from build123d import *

# Parameters (mm, degrees)
SKETCH2_W           = 48.13
SKETCH2_H           = 41.71
BOSS_EXTRUDE1_DEPTH = 1.71
SKETCH3_R           = 1.5
CUT_EXTRUDE1_DEPTH  = 10.71
CUT_EXTRUDE2_DEPTH  = 10.71
FILLET3_R           = 2.5
SKETCH8_W           = 8.21
SKETCH8_H           = 30.23
BOSS_EXTRUDE2_DEPTH = 10.03


with BuildPart() as part:
    # Sketch2 → Boss-Extrude1 (new body)
    with BuildSketch(Plane(origin=(0, 0, 0), x_dir=(1, 0, 0), z_dir=(0, 1, 0))):
        Rectangle(SKETCH2_W, SKETCH2_H)
    extrude(amount=BOSS_EXTRUDE1_DEPTH)

    # Sketch3 → Cut-Extrude1 (cut)
    with BuildSketch(Plane(origin=(0, 1.71, 0), x_dir=(1, 0, 0), z_dir=(0, 1, 0))):
        with Locations(Location((-21.545702182, 18.174313444, 0), (0, 0, 270))):
            Circle(SKETCH3_R)
    cut_extrude1 = extrude(amount=-CUT_EXTRUDE1_DEPTH, mode=Mode.SUBTRACT)

    # Sketch4 → Cut-Extrude2 (cut)
    with BuildSketch(Plane(origin=(0, 1.71, 0), x_dir=(1, 0, 0), z_dir=(0, 1, 0))):
        with BuildLine():
            ThreePointArc((-20.045702182, -18.175), (-20.485042011, -17.114339828), (-21.545702182, -16.675))
            Line((-21.545702182, -16.675), (-21.545702182, -18.175))
            Line((-21.545702182, -18.175), (-21.545702182, -19.675))
            ThreePointArc((-21.545702182, -19.675), (-20.485042011, -19.235660172), (-20.045702182, -18.175))
        make_face()
        with BuildLine():
            Line((-21.545702182, -18.175), (-21.545702182, -16.675))
            ThreePointArc((-21.545702182, -16.675), (-23.045702182, -18.175), (-21.545702182, -19.675))
            Line((-21.545702182, -19.675), (-21.545702182, -18.175))
        make_face()
    cut_extrude2 = extrude(amount=-CUT_EXTRUDE2_DEPTH, mode=Mode.SUBTRACT)

    # Fillet3
    fillet3_edges = [part.edges().sort_by_distance(p)[0] for p in [
        (24.065, 0.855, 20.855),
        (-24.065, 0.855, 20.855),
        (-24.065, 0.855, -20.855),
        (24.065, 0.855, -20.855),
    ]]
    fillet(fillet3_edges, radius=FILLET3_R)

    # Mirror1: Cut-Extrude1, Cut-Extrude2 across plane
    add(cut_extrude1.mirror(Plane(origin=(0, 0, 0), x_dir=(0, 0, 1), z_dir=(1, 0, 0))), mode=Mode.SUBTRACT)
    add(cut_extrude2.mirror(Plane(origin=(0, 0, 0), x_dir=(0, 0, 1), z_dir=(1, 0, 0))), mode=Mode.SUBTRACT)

    # Sketch8 → Boss-Extrude2 (add)
    with BuildSketch(Plane(origin=(0, 1.71, 0), x_dir=(1, 0, 0), z_dir=(0, 1, 0))):
        with Locations((-19.96, 0)):
            Rectangle(SKETCH8_W, SKETCH8_H)
    extrude(amount=BOSS_EXTRUDE2_DEPTH)


solid = part.part
The listing builds one solid part. Answer for the finished solid, in the listing's coordinates (mm). A direction names the side the tool comes from. Round coordinates to 2 decimals unless told otherwise and drop trailing zeros. Order: outer loops, then holes, each group sorted by start corner. A loop starts at its lowest first (then second) coordinate and runs counter-clockwise, first axis right, second up. Notation, with made-up numbers: M 8.5,-21 L 35.5,-21 A18 cw 35.5,-13 Z; hole C -35.75,86 d9. An arc over 180 degrees is marked long. Answer in a Markdown table with one row per item. Add a question column.
1) The part is cut by section B-B on z = 13. Determine the outline of the cut face in (x, y) (3 decimals).
2) The part is cut by section A-A on x = -21. Determine the outline of the cut face in (y, z) (3 decimals), plus the area to 3 significant figures.
3) The part is cut by section D-D on x = 12.5. Determine the outline of the cut face in (y, z) (3 decimals).
4) Flat-ended cylindrical pins translate along their axes: pin 1 Ø5 at (x, z) = (21.55, -18.17) entering from +Y; pin 2 Ø6 at (y, z) = (4.5, 12) entering from +X (3 decimals); pin 3 Ø2.5 at (x, z) = (-21.55, -18.17) entering from +Y; pin 4 Ø2.5 at (x, y) = (-18, 5.5) entering from +Z (3 decimals). Find the tip coordinate at first contact, or state that the pin passes through.
5) The part is cut by section C-C on y = 7.25. Determine the outline of the cut face in (x, z) (3 decimals), plus the area to 3 significant figures.
6) Consider line 1 along Z through (x, y) = (-20.5, 1.5) (3 decimals); line 2 along Y through (x, z) = (17, -4); line 3 along X through (y, z) = (2, -15) (3 decimals). Determine where each line is inside the solid, lowest interval first. Write a range as from..to.
7) Determine the mould class of faces 1 (the face through (0, 0, 0)), 2 (the face through (0, 1, 20.855)), 3 (the face through (-21.48, 0.867, -19.673)) for opening direction Z: pulls with the +Z half, pulls with the -Z half, needs draft (parallel to the pull), parting line crosses it, or undercut.
8) Which of the six approach directions +Z, -Z, +X, -X, +Y, -Y give full straight-line access (tool end or side, diameter ignored) to faces 4 (the face through (-15.855, 7, 0)), 5 (the face through (-20, 7, 15.115)), 6 (the face through (-20, 7, -15.115))?
Findings below:
| question | item | result |
|---|---|---|
| 1 | outline | M -24.065,0 L 24.065,0 L 24.065,1.71 L -15.855,1.71 L -15.855,11.74 L -24.065,11.74 Z |
| 2 | outline | M 0,-20.855 L 1.71,-20.855 L 1.71,-19.572 L 0,-19.572 Z; M 0,-16.777 L 1.71,-16.777 L 1.71,-15.115 L 11.74,-15.115 L 11.74,15.115 L 1.71,15.115 L 1.71,16.778 L 0,16.778 Z; M 0,19.572 L 1.71,19.572 L 1.71,20.855 L 0,20.855 Z |
| 2 | area | 365 mm² |
| 3 | outline | M 0,-20.855 L 1.71,-20.855 L 1.71,20.855 L 0,20.855 Z |
| 4 | pin 1 | stops at y = 1.71 |
| 4 | pin 2 | stops at x = 24.065 |
| 4 | pin 3 | passes through |
| 4 | pin 4 | stops at z = 15.115 |
| 5 | outline | M -24.065,-15.115 L -15.855,-15.115 L -15.855,15.115 L -24.065,15.115 Z |
| 5 | area | 248 mm² |
| 6 | line 1 | z = -20.855..-19.25, -17.099..17.1, 19.25..20.855 |
| 6 | line 2 | y = 0..1.71 |
| 6 | line 3 | x = -24.065..-15.855 |
| 7 | face 1 | needs draft |
| 7 | face 2 | pulls with the +Z half |
| 7 | face 3 | undercut |
| 8 | face 4 | +Z, -Z, +X, +Y |
| 8 | face 5 | +Z, +X, -X, +Y |
| 8 | face 6 | -Z, +X, -X, +Y |
